Part print with two shaded views. Sizes in mm from the minimum x, y, z corner. Give positions to 0.01 mm unless a question says otherwise; leave off trailing zeros. Order: outer loops, then holes, each group sorted by start corner. A loop starts at its lowest first (then second) coordinate and runs counter-clockwise, first axis right, second up. Notation, with made-up numbers: (31, -11.5) -> (71, -11.5) arc R24 ccw to (71, 15.5) -> close; hole circle Ø2 at (-15, -35). An arc over 180 degrees is marked (long way). Write item = value, one per line. Start each with the question number.
Item 1: Band-saw the part on D-D on y = 6. Write the cut outline in (x, z).
Item 2: Pull direction Y, two halves, no side cores. Call the marked faces 1, 2, 3 and 4: +Y half, -Y half, draft (parallel to the pull), parting line (faces both ways), or undercut.
Item 3: Drill centre lines: line 1 along Y through (x, z) = (34.5, 1.5); line 2 along X through (y, z) = (2.5, 2.15) (1 decimal); line 3 along Y through (x, z) = (13, 2.6). Where is each one in solid material? Low to high.
Item 4: Flat gauge pin, fed straight in: P1, Ø1, axis at y = 5.5, z = 2, coming from the +X side. Where does the tip first touch, or does it go through?
Item 5: Band-saw the part on B-B on z = 2.7. Write the cut outline in (x, y) (1 decimal), plus the area to 3 significant figures.
Item 6: Band-saw the part on C-C on y = 4. Write the cut outline in (x, z), plus the area to 3 significant figures.
Item 7: Band-saw the part on A-A on x = 3.5. Write the cut outline in (y, z).
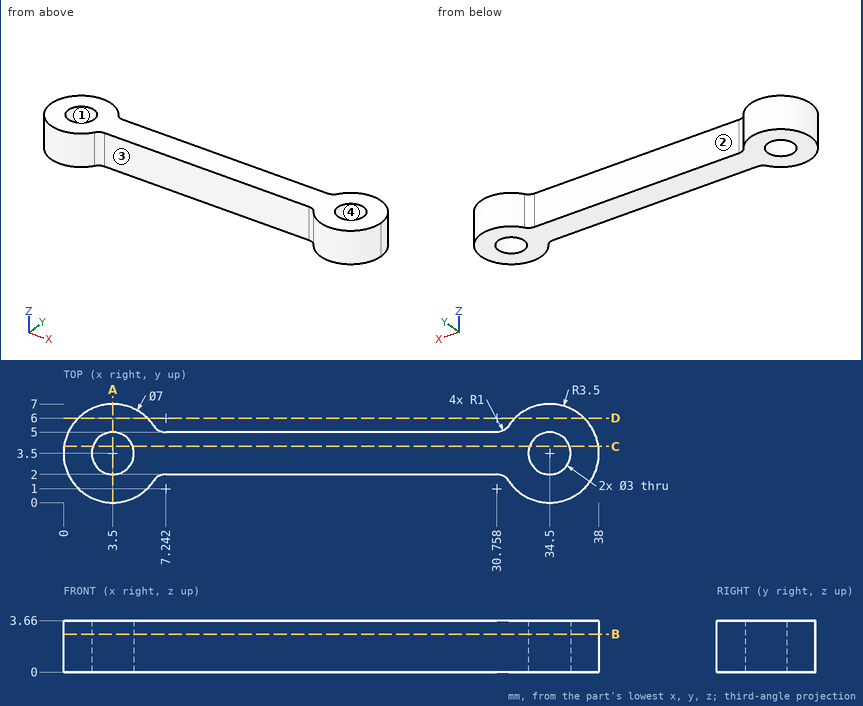
Values found:
q1.outline = (1.05, 0) -> (5.95, 0) -> (5.95, 3.66) -> (1.05, 3.66) -> close; (32.05, 0) -> (36.95, 0) -> (36.95, 3.66) -> (32.05, 3.66) -> close
q2.face_1 = undercut
q2.face_2 = +Y half
q2.face_3 = -Y half
q2.face_4 = undercut
q3.line_1 = 0 to 2, 5 to 7
q3.line_2 = 0.1 to 2.4, 4.6 to 33.4, 35.6 to 37.9
q3.line_3 = 2 to 5
q4.P1 = 37.66
q5.outline = (6.4, 1.6) arc R1 cw to (7.2, 2) -> (30.8, 2) arc R1 cw to (31.6, 1.6) arc R3.5 ccw (long way) to (31.6, 5.4) arc R1 cw to (30.8, 5) -> (7.2, 5) arc R1 cw to (6.4, 5.4) arc R3.5 ccw (long way) to start; hole circle Ø3 at (3.5, 3.5); hole circle Ø3 at (34.5, 3.5)
q5.area = 136 mm^2
q6.outline = (0.04, 0) -> (2.09, 0) -> (2.09, 3.66) -> (0.04, 3.66) -> close; (4.91, 0) -> (33.09, 0) -> (33.09, 3.66) -> (4.91, 3.66) -> close; (35.91, 0) -> (37.96, 0) -> (37.96, 3.66) -> (35.91, 3.66) -> close
q6.area = 118 mm^2
q7.outline = (0, 0) -> (2, 0) -> (2, 3.66) -> (0, 3.66) -> close; (5, 0) -> (7, 0) -> (7, 3.66) -> (5, 3.66) -> close
